from build123d import *

# Parameters (mm, degrees)
F0_R     = 10.795
F1_DEPTH = 25.4
F3_DEPTH = 25.401
F4_DEPTH = 11.0998


with BuildPart() as f1:
    # F0 (on Front) → F1 (new body)
    with BuildSketch(Plane.XZ):
        Circle(F0_R)
    extrude(amount=F1_DEPTH)

    # F2 (on Front) → F3 (cut, through all)
    with BuildSketch(Plane.XZ):
        with BuildLine():
            ThreePointArc((4.7625, 0), (3.367596, 3.367596), (0, 4.7625))
            ThreePointArc((0, 4.7625), (-3.367596, 3.367596), (-4.7625, 0))
            ThreePointArc((-4.7625, 0), (-3.367596, -3.367596), (0, -4.7625))
            ThreePointArc((0, -4.7625), (3.367596, -3.367596), (4.7625, 0))
        make_face()
    extrude(amount=F3_DEPTH, mode=Mode.SUBTRACT)

    # F2 (on Front) → F4 (cut)
    with BuildSketch(Plane.XZ):
        with BuildLine():
            Line((4.7625, 0), (4.7625, 4.7625))
            Line((4.7625, 4.7625), (0, 4.7625))
            ThreePointArc((0, 4.7625), (3.367596, 3.367596), (4.7625, 0))
        make_face()
        with BuildLine():
            ThreePointArc((-4.7625, 0), (-3.367596, 3.367596), (0, 4.7625))
            Line((0, 4.7625), (-4.7625, 4.7625))
            Line((-4.7625, 4.7625), (-4.7625, 0))
        make_face()
        with BuildLine():
            Line((4.7625, -4.7625), (4.7625, 0))
            ThreePointArc((4.7625, 0), (3.367596, -3.367596), (0, -4.7625))
            Line((0, -4.7625), (4.7625, -4.7625))
        make_face()
        with BuildLine():
            ThreePointArc((0, -4.7625), (-3.367596, -3.367596), (-4.7625, 0))
            Line((-4.7625, 0), (-4.7625, -4.7625))
            Line((-4.7625, -4.7625), (0, -4.7625))
        make_face()
    extrude(amount=F4_DEPTH, mode=Mode.SUBTRACT)


solid = f1.part
Can you work these out from the model? Positions are in its coordinate system, mm. A direction names the side the tool comes from. Give positions to 0.01 mm unless a question says otherwise; leave off trailing zeros. Loops run counter-clockwise (first coordinate to the right, second up) from the corner with the lowest first, then second, coordinate; pieces in that order, holes last. Notation, with made-up numbers: (-19.5, -22.75) -> (-10.5, -22.75) arc R19 cw to (-10.5, -8.75) -> close; hole circle Ø1 at (76, 3.5). An arc over 180 degrees is marked (long way). Use one line per item in the form item = value.
1) I need wall thicknesses on line 1 along Z through (x, y) = (0.25, -20.25); line 2 along X through (y, z) = (-15.75, 3.5); line 3 along X through (y, z) = (-11, 1.5). Which ranges of each line are inside material? Lowest first, please.
Answers:
line_1 = -10.79 to -4.76, 4.76 to 10.79
line_2 = -10.21 to -3.23, 3.23 to 10.21
line_3 = -10.69 to -4.76, 4.76 to 10.69
2) If we section it at B-B (x = -2): Please give me the cut outline in (y, z), plus the area to 3 significant figures.
Answers:
outline = (-25.4, -10.61) -> (0, -10.61) -> (0, -4.76) -> (-11.1, -4.76) -> (-11.1, -4.32) -> (-25.4, -4.32) -> close; (-25.4, 4.32) -> (-11.1, 4.32) -> (-11.1, 4.76) -> (0, 4.76) -> (0, 10.61) -> (-25.4, 10.61) -> close
area = 310 mm²
3) If we section it at A-A (z = -1.75): Please give me the cut outline in (x, y).
Answers:
outline = (-10.65, -25.4) -> (-4.43, -25.4) -> (-4.43, -11.1) -> (-4.76, -11.1) -> (-4.76, 0) -> (-10.65, 0) -> close; (4.43, -25.4) -> (10.65, -25.4) -> (10.65, 0) -> (4.76, 0) -> (4.76, -11.1) -> (4.43, -11.1) -> close
4) For faces 1 (the face through (-5, 0, 0)), 2 (the face through (-4, -11.1, -4)), which set-ups out of +Z, -Z, +X, -X, +Y, -Y let a thin tool reach every point of the face, with its end or its side?
Answers:
face_1 = +Z, -Z, +X, -X, +Y
face_2 = +Y
5) We'd pull the mould along X, two halves only. Please class faces 3 (the face through (-7.956, -12.522, 7.296)), 4 (the face through (4, -11.1, -4)), 5 (the face through (5, -25.4, -2)): released by +X, released by -X, zero draft, split by the parting line, or undercut.
Answers:
face_3 = split by the parting line
face_4 = undercut
face_5 = zero draft
6) If we section it at C-C (y = -22.5): Please give me the cut outline in (x, z) (1 decimal), plus the area to 3 significant figures.
Answers:
outline = circle Ø21.6 at (0, 0); hole circle Ø9.5 at (0, 0)
area = 295 mm²
7) Will these pins go through, and if not, where does the flat tip stop? pin 1 (2 mm diameter, centred on y = -13, z = -8, fed in from -X); pin 2 (12 mm diameter, centred on y = -5.5, z = -8, fed in from -X); pin 3 (5 mm diameter, centred on x = 5, y = -10, fed in from +Z).
Answers:
pin_1 = -8.22
pin_2 = -10.61
pin_3 = 10.5
8) If we section it at D-D (y = -5): Please give me the cut outline in (x, z) (1 decimal).
Answers:
outline = circle Ø21.6 at (0, 0); hole (-4.8, -4.8) -> (4.8, -4.8) -> (4.8, 4.8) -> (-4.8, 4.8) -> close
